```python
from build123d import *

# Parameters (mm, degrees)
F1_DEPTH = 260


# Not quite as in the source:
# - ends of sketch curves that miss each other by under 0.0002 mm in the source are joined


with BuildPart() as f1:
    # F0 (on Front) → F1 (new body)
    with BuildSketch(Plane.XZ):
        with BuildLine():
            ThreePointArc((-2.15, 0), (-1.5202795796, 1.5202795796), (0, 2.15))
            Line((0, 2.15), (0, 3))
            Line((0, 3), (-0.307277, 3.307278))
            ThreePointArc((-0.307277, 3.307278), (-2.2820211583, 3.7143800615), (-4.036565823, 4.7078182229))
            ThreePointArc((-4.036565823, 4.7078182229), (-4.1201572004, 4.8123081084), (-4.15, 4.94275))
            Line((-4.15, 4.94275), (-4.15, 8.2))
            ThreePointArc((-4.15, 8.2), (-4.0621320344, 8.4121320344), (-3.85, 8.5))
            Line((-3.85, 8.5), (-2.95, 8.5))
            ThreePointArc((-2.95, 8.5), (-2.7378679656, 8.5878679656), (-2.65, 8.8))
            Line((-2.65, 8.8), (-2.65, 9.7))
            ThreePointArc((-2.65, 9.7), (-2.7378679656, 9.9121320344), (-2.95, 10))
            Line((-2.95, 10), (-9.7, 10))
            ThreePointArc((-9.7, 10), (-9.9121320344, 9.9121320344), (-10, 9.7))
            Line((-10, 9.7), (-10, 2.95))
            ThreePointArc((-10, 2.95), (-9.9121320344, 2.7378679656), (-9.7, 2.65))
            Line((-9.7, 2.65), (-8.8, 2.65))
            ThreePointArc((-8.8, 2.65), (-8.5878679656, 2.7378679656), (-8.5, 2.95))
            Line((-8.5, 2.95), (-8.5, 3.85))
            ThreePointArc((-8.5, 3.85), (-8.4121320344, 4.0621320344), (-8.2, 4.15))
            Line((-8.2, 4.15), (-4.942749, 4.15))
            ThreePointArc((-4.942749, 4.15), (-4.812307461, 4.1201573706), (-4.7078173786, 4.0365666993))
            ThreePointArc((-4.7078173786, 4.0365666993), (-3.7143793747, 2.2820219924), (-3.3072773955, 0.3072779813))
            Line((-3.3072773955, 0.3072779813), (-3, 0))
            Line((-3, 0), (-2.15, 0))
        make_face()
        with BuildLine():
            ThreePointArc((-7, 5), (-8.4142135624, 5.5857864376), (-9, 7))
            ThreePointArc((-9, 7), (-8.4142135624, 8.4142135624), (-7, 9))
            ThreePointArc((-7, 9), (-5.5857864376, 8.4142135624), (-5, 7))
            ThreePointArc((-5, 7), (-5.5857864376, 5.5857864376), (-7, 5))
        make_face(mode=Mode.SUBTRACT)
        with BuildLine():
            ThreePointArc((0, 2.15), (1.5202795796, 1.5202795796), (2.15, 0))
            Line((2.15, 0), (3, 0))
            Line((3, 0), (3.307278, 0.307278))
            ThreePointArc((3.307278, 0.307278), (3.7143803747, 2.2820219924), (4.7078187099, 4.0365664363))
            ThreePointArc((4.7078187099, 4.0365664363), (4.812308461, 4.1201573706), (4.94275, 4.15))
            Line((4.94275, 4.15), (8.2, 4.15))
            ThreePointArc((8.2, 4.15), (8.4121320344, 4.0621320344), (8.5, 3.85))
            Line((8.5, 3.85), (8.5, 2.95))
            ThreePointArc((8.5, 2.95), (8.5878679656, 2.7378679656), (8.8, 2.65))
            Line((8.8, 2.65), (9.7, 2.65))
            ThreePointArc((9.7, 2.65), (9.9121320344, 2.7378679656), (10, 2.95))
            Line((10, 2.95), (10, 9.7))
            ThreePointArc((10, 9.7), (9.9121320344, 9.9121320344), (9.7, 10))
            Line((9.7, 10), (2.95, 10))
            ThreePointArc((2.95, 10), (2.7378679656, 9.9121320344), (2.65, 9.7))
            Line((2.65, 9.7), (2.65, 8.8))
            ThreePointArc((2.65, 8.8), (2.7378679656, 8.5878679656), (2.95, 8.5))
            Line((2.95, 8.5), (3.85, 8.5))
            ThreePointArc((3.85, 8.5), (4.0621320344, 8.4121320344), (4.15, 8.2))
            Line((4.15, 8.2), (4.15, 4.94275))
            ThreePointArc((4.15, 4.94275), (4.1201572004, 4.8123081084), (4.036566086, 4.7078178916))
            ThreePointArc((4.036566086, 4.7078178916), (2.2820216259, 3.7143802371), (0.3072779813, 3.3072783955))
            Line((0.3072779813, 3.3072783955), (0, 3))
            Line((0, 3), (0, 2.15))
        make_face()
        with BuildLine():
            ThreePointArc((7, 9), (8.4142135624, 8.4142135624), (9, 7))
            ThreePointArc((9, 7), (8.4142135624, 5.5857864376), (7, 5))
            ThreePointArc((7, 5), (5.5857864376, 5.5857864376), (5, 7))
            ThreePointArc((5, 7), (5.5857864376, 8.4142135624), (7, 9))
        make_face(mode=Mode.SUBTRACT)
        with BuildLine():
            Line((3, 0), (2.15, 0))
            ThreePointArc((2.15, 0), (1.5202795796, -1.5202795796), (0, -2.15))
            Line((0, -2.15), (0, -3))
            Line((0, -3), (0.307278, -3.307277))
            ThreePointArc((0.307278, -3.307277), (2.2820216259, -3.7143792371), (4.036565823, -4.7078172229))
            ThreePointArc((4.036565823, -4.7078172229), (4.1201572004, -4.8123071084), (4.15, -4.942749))
            Line((4.15, -4.942749), (4.15, -8.2))
            ThreePointArc((4.15, -8.2), (4.0621320344, -8.4121320344), (3.85, -8.5))
            Line((3.85, -8.5), (2.95, -8.5))
            ThreePointArc((2.95, -8.5), (2.7378679656, -8.5878679656), (2.65, -8.8))
            Line((2.65, -8.8), (2.65, -9.7))
            ThreePointArc((2.65, -9.7), (2.7378679656, -9.9121320344), (2.95, -10))
            Line((2.95, -10), (9.7, -10))
            ThreePointArc((9.7, -10), (9.9121320344, -9.9121320344), (10, -9.7))
            Line((10, -9.7), (10, -2.95))
            ThreePointArc((10, -2.95), (9.9121320344, -2.7378679656), (9.7, -2.65))
            Line((9.7, -2.65), (8.8, -2.65))
            ThreePointArc((8.8, -2.65), (8.5878679656, -2.7378679656), (8.5, -2.95))
            Line((8.5, -2.95), (8.5, -3.85))
            ThreePointArc((8.5, -3.85), (8.4121320344, -4.0621320344), (8.2, -4.15))
            Line((8.2, -4.15), (4.94275, -4.15))
            ThreePointArc((4.94275, -4.15), (4.8123081084, -4.1201572004), (4.7078178916, -4.036566086))
            ThreePointArc((4.7078178916, -4.036566086), (3.7143800615, -2.2820211583), (3.3072783483, -0.3072769835))
            Line((3.3072783483, -0.3072769835), (3, 0))
        make_face()
        with BuildLine():
            ThreePointArc((7, -5), (8.4142135624, -5.5857864376), (9, -7))
            ThreePointArc((9, -7), (8.4142135624, -8.4142135624), (7, -9))
            ThreePointArc((7, -9), (5.5857864376, -8.4142135624), (5, -7))
            ThreePointArc((5, -7), (5.5857864376, -5.5857864376), (7, -5))
        make_face(mode=Mode.SUBTRACT)
        with BuildLine():
            Line((0, -3), (0, -2.15))
            ThreePointArc((0, -2.15), (-1.5202795796, -1.5202795796), (-2.15, 0))
            Line((-2.15, 0), (-3, 0))
            Line((-3, 0), (-3.307277, -0.307277))
            ThreePointArc((-3.307277, -0.307277), (-3.7143790615, -2.2820211583), (-4.7078172229, -4.036565823))
            ThreePointArc((-4.7078172229, -4.036565823), (-4.8123071084, -4.1201572004), (-4.942749, -4.15))
            Line((-4.942749, -4.15), (-8.2, -4.15))
            ThreePointArc((-8.2, -4.15), (-8.4121320344, -4.0621320344), (-8.5, -3.85))
            Line((-8.5, -3.85), (-8.5, -2.95))
            ThreePointArc((-8.5, -2.95), (-8.5878679656, -2.7378679656), (-8.8, -2.65))
            Line((-8.8, -2.65), (-9.7, -2.65))
            ThreePointArc((-9.7, -2.65), (-9.9121320344, -2.7378679656), (-10, -2.95))
            Line((-10, -2.95), (-10, -9.7))
            ThreePointArc((-10, -9.7), (-9.9121320344, -9.9121320344), (-9.7, -10))
            Line((-9.7, -10), (-2.95, -10))
            ThreePointArc((-2.95, -10), (-2.7378679656, -9.9121320344), (-2.65, -9.7))
            Line((-2.65, -9.7), (-2.65, -8.8))
            ThreePointArc((-2.65, -8.8), (-2.7378679656, -8.5878679656), (-2.95, -8.5))
            Line((-2.95, -8.5), (-3.85, -8.5))
            ThreePointArc((-3.85, -8.5), (-4.0621320344, -8.4121320344), (-4.15, -8.2))
            Line((-4.15, -8.2), (-4.15, -4.942749))
            ThreePointArc((-4.15, -4.942749), (-4.1201572004, -4.8123071084), (-4.036566086, -4.7078168916))
            ThreePointArc((-4.036566086, -4.7078168916), (-2.2820211583, -3.7143790615), (-0.3072769835, -3.3072773483))
            Line((-0.3072769835, -3.3072773483), (0, -3))
        make_face()
        with BuildLine():
            ThreePointArc((-7, -9), (-8.4142135624, -8.4142135624), (-9, -7))
            ThreePointArc((-9, -7), (-8.4142135624, -5.5857864376), (-7, -5))
            ThreePointArc((-7, -5), (-5.5857864376, -5.5857864376), (-5, -7))
            ThreePointArc((-5, -7), (-5.5857864376, -8.4142135624), (-7, -9))
        make_face(mode=Mode.SUBTRACT)
    extrude(amount=F1_DEPTH)


solid = f1.part
```
The model under review builds one solid part; all positions refer to its coordinate system, in mm. Round coordinates to 2 decimals unless told otherwise and drop trailing zeros. Answer in a Markdown table with one row per item.
(1) Clearance check with flat-ended pins moving along their axes: P1, Ø2, axis at x = 0, z = 1, coming from the +Y side; P2, Ø2, axis at x = -0.5, y = -232.5, coming from the -Z side. State where each tip first meets the part, or that it passes through.
Result set:
| item | result |
|---|---|
| P1 | passes through |
| P2 | stops at z = -3.48 |
(2) For line 1 (X direction, y = -226.5, z = 4); line 2 (X direction, y = -186.5, z = 7.25), list the stretches that pass through material, from the lowest coordinate up. Write a range as from..to.
Result set:
| item | result |
|---|---|
| line 1 | x = -10..-8.46, -4.68..-2.93, 2.93..4.68, 8.46..10 |
| line 2 | x = -10..-8.98, -5.02..-4.15, 4.15..5.02, 8.98..10 |
(3) Mouldability with a two-part tool opening along Y and no side actions: class faces 1 (the face through (10, -128, 6)), 2 (the face through (-2.4, -260, 0.1)), 3 (the face through (-2.4, 0, 0.1)) as released by +Y, released by -Y, zero draft, split by the parting line, or undercut.
Result set:
| item | result |
|---|---|
| face 1 | zero draft |
| face 2 | released by -Y |
| face 3 | released by +Y |
(4) Take a section at A-A on y = -91. Count the separate pieces of the cut face and the enclosed holes in it, plus the area to 3 significant figures.
Result set:
| item | result |
|---|---|
| separate pieces | 1 |
| enclosed holes | 5 |
| area | 146 mm2 |
